Geometry: final body of the model. Coordinates: model frame, mm. A direction names the side the tool comes from. Give positions to 0.01 mm unless a question says otherwise; leave off trailing zeros. Write each loop counter-clockwise with the first axis right and the second up, starting at its lowest first coordinate (ties: lowest second). Pieces come first, ordered by that corner, then holes. Notation, with made-up numbers: M -3.75,6 L 11.25,6 A28 ccw 11.25,28 Z; hole C -9.75,53 d1. An arc over 180 degrees is marked long. Use a Markdown table: item, result. Add a question column.
1) Section B-B on z = -70.5. Return the cut outline in (x, y).
2) Section D-D on y = 26. Return the cut outline in (x, z), then the cut area to 3 significant figures.
3) Pin query (flat end, axial travel): pin 1 (3 mm diameter, centred on x = 128, y = 3.5, fed in from +Z); pin 2 (5 mm diameter, centred on y = 13, z = -29.5, fed in from +X); pin 3 (2 mm diameter, centred on y = 60, z = -17.5, fed in from -X); pin 4 (11 mm diameter, centred on x = 157.5, y = 5, fed in from -Z). Return the tip coordinate at first contact, or that it passes through.
4) Line query: line 1 (X direction, y = 14, z = 0); line 2 (Z direction, x = 198, y = 66.5); line 3 (X direction, y = 4.5, z = 0). Output: solid intervals per line, ascending.
5) Section A-A on x = 0. State how many separate pieces and enclosed holes the cut face has, then the cut area to 3 significant figures.
6) Set-up query: faces 5 (the flat face through (198, 53.3, -11)), 6 (the flat face through (214, 72, 0)), 7 (the flat face through (217.05, 62, 0)), 8 (the cylindrical face through (223.3, 4.93, -3.06)), 9 (the cylindrical face through (-46.245, 14.93, -60.311)). Return all of +Z, -Z, +X, -X, +Y, -Y with unobstructed straight access to the full face (end or side cutting, diameter ignored); none if empty.
7) Draft query along Y for faces 1 (the flat face through (187, 80, 0)), 2 (the flat face through (-57.5, 20, 19)), 3 (the flat face through (190, 63, -15)), 4 (the cylindrical face through (-66.284, 5.07, 2.688)). Return one class per face: +Y half, -Y half, draft (parallel to the pull), parting line (faces both ways), or undercut.
8) Section C-C on x = -70.5. Return the cut outline in (y, z).
```python
from build123d import *

# Parameters (mm, degrees)
CROQUIS1_R                   = 50
CROQUIS1_R_2                 = 23.5
SALIENTE_EXTRUIR1_DEPTH      = 10
REDONDEO1_R                  = 70
CROQUIS2_R                   = 81
CROQUIS2_R_2                 = 76
SALIENTE_EXTRUIR2_DEPTH      = 10
CROQUIS8_W                   = 74
CROQUIS8_H                   = 10
SALIENTE_EXTRUIR4_DEPTH      = 10
CROQUIS9_W                   = 74
CROQUIS9_H                   = 10
SALIENTE_EXTRUIR5_DEPTH      = 80
CROQUIS10_W                  = 74
CROQUIS10_H                  = 10
SALIENTE_EXTRUIR6_DEPTH      = 75
REDONDEO3_R                  = 2
REDONDEO4_R                  = 2
REDONDEO5_R                  = 2
REDONDEO6_R                  = 2
CROQUIS12_R                  = 65
CROQUIS12_R_2                = 60
SALIENTE_EXTRUIR12_DEPTH     = 10
CROQUIS13_R                  = 5
CORTAR_EXTRUIR1_DEPTH        = 10
SALIENTE_EXTRUIR13_OUTLINE_R = 1.25
SALIENTE_EXTRUIR13_DEPTH     = 26.7
REDONDEO7_R                  = 10
CORTAR_EXTRUIR2_START        = -36.7
CROQUIS15_R                  = 1.25
CORTAR_EXTRUIR2_DEPTH        = 36.7
REDONDEO9_R                  = 2.5
CROQUIS17_W                  = 7
CROQUIS17_H                  = 5
CORTAR_EXTRUIR3_DEPTH        = 26.95
CROQUIS18_W                  = 40.143208987
CROQUIS18_H                  = 75
CORTAR_EXTRUIR4_DEPTH        = 5
REDONDEO10_R                 = 1
REDONDEO11_R                 = 1


# Read off the part's stored shape, not the designer's step: Saliente-Extruir13
with BuildPart() as part:
    # Croquis1 → Saliente-Extruir1 (new body)
    with BuildSketch(Plane(origin=(0, 0, 0), x_dir=(1, 0, 0), z_dir=(0, 1, 0))):
        with BuildLine():
            ThreePointArc((-72.570488149, -44.255217205), (4.131356705, -84.899539997), (76.524505879, -37))
            Line((76.524505879, -37), (237, -37))
            Line((237, -37), (237, 0))
            ThreePointArc((237, 0), (226.162950904, 26.162950904), (200, 37))
            Line((200, 37), (76.524505879, 37))
            ThreePointArc((76.524505879, 37), (4.131356705, 84.899539997), (-72.570488149, 44.255217205))
            Line((-72.570488149, 44.255217205), (-135.143208987, 44.255217205))
            Line((-135.143208987, 44.255217205), (-135.143208987, -44.255217205))
            Line((-135.143208987, -44.255217205), (-72.570488149, -44.255217205))
        make_face()
        with Locations(Location((0, 0, 0), (0, 0, 270))):
            Circle(CROQUIS1_R, mode=Mode.SUBTRACT)
        with Locations(Location((200, 0, 0), (0, 0, 270))):
            Circle(CROQUIS1_R_2, mode=Mode.SUBTRACT)
    extrude(amount=SALIENTE_EXTRUIR1_DEPTH)

    # Redondeo1
    redondeo1_edges = [part.edges().sort_by_distance(p)[0] for p in [
        (76.524505879, 5, 37),
        (-72.570488149, 5, 44.255217205),
        (-72.570488149, 5, -44.255217205),
        (76.524505879, 5, -37),
    ]]
    fillet(redondeo1_edges, radius=REDONDEO1_R)

    # Croquis2 → Saliente-Extruir2 (add)
    with BuildSketch(Plane(origin=(0, 10, 0), x_dir=(1, 0, 0), z_dir=(0, 1, 0))):
        with Locations(Location((0, 0, 0), (0, 0, 270))):
            Circle(CROQUIS2_R)
        with Locations(Location((0, 0, 0), (0, 0, 270))):
            Circle(CROQUIS2_R_2, mode=Mode.SUBTRACT)
    extrude(amount=SALIENTE_EXTRUIR2_DEPTH)

    # Croquis8 → Saliente-Extruir4 (add)
    with BuildSketch(Plane.XY.offset(37)):
        with Locations((200, 5)):
            Rectangle(CROQUIS8_W, CROQUIS8_H)
    extrude(amount=SALIENTE_EXTRUIR4_DEPTH)

    # Croquis9 → Saliente-Extruir5 (add)
    with BuildSketch(Plane(origin=(0, 10, 0), x_dir=(1, 0, 0), z_dir=(0, 1, 0))):
        with Locations((200, -42)):
            Rectangle(CROQUIS9_W, CROQUIS9_H)
    extrude(amount=SALIENTE_EXTRUIR5_DEPTH)

    # Croquis10 → Saliente-Extruir6 (add)
    with BuildSketch(Plane(origin=(0, 0, 37), x_dir=(-1, 0, 0), z_dir=(0, 0, -1))):
        with Locations((-200, 85)):
            Rectangle(CROQUIS10_W, CROQUIS10_H)
    extrude(amount=SALIENTE_EXTRUIR6_DEPTH)

    # Redondeo3
    redondeo3_edges = [part.edges().sort_by_distance(p)[0] for p in [
        (200, 10, 37),
    ]]
    fillet(redondeo3_edges, radius=REDONDEO3_R)

    # Redondeo4
    redondeo4_edges = [part.edges().sort_by_distance(p)[0] for p in [
        (200, 80, 37),
    ]]
    fillet(redondeo4_edges, radius=REDONDEO4_R)

    # Redondeo5
    redondeo5_edges = [part.edges().sort_by_distance(p)[0] for p in [
        (200, 90, 47),
    ]]
    fillet(redondeo5_edges, radius=REDONDEO5_R)

    # Redondeo6
    redondeo6_edges = [part.edges().sort_by_distance(p)[0] for p in [
        (200, 90, -38),
    ]]
    fillet(redondeo6_edges, radius=REDONDEO6_R)

    # Croquis12 → Saliente-Extruir12 (add)
    with BuildSketch(Plane(origin=(0, 10, 0), x_dir=(1, 0, 0), z_dir=(0, 1, 0))):
        with Locations(Location((0, 0, 0), (0, 0, 270))):
            Circle(CROQUIS12_R)
        with Locations(Location((0, 0, 0), (0, 0, 270))):
            Circle(CROQUIS12_R_2, mode=Mode.SUBTRACT)
    extrude(amount=SALIENTE_EXTRUIR12_DEPTH)

    # Croquis13 → Cortar-Extruir1 (cut)
    with BuildSketch(Plane(origin=(0, 10, 0), x_dir=(1, 0, 0), z_dir=(0, 1, 0))):
        with Locations(Location((-70.5, 0, 0), (0, 0, 270))):
            Circle(CROQUIS13_R)
        with Locations(Location((0, 70.5, 0), (0, 0, 270))):
            Circle(CROQUIS13_R)
        with Locations(Location((70.5, 0, 0), (0, 0, 270))):
            Circle(CROQUIS13_R)
        with Locations(Location((0, -70.5, 0), (0, 0, 270))):
            Circle(CROQUIS13_R)
    extrude(amount=-CORTAR_EXTRUIR1_DEPTH, mode=Mode.SUBTRACT)

    # Saliente-Extruir13 outline → Saliente-Extruir13 (add)
    with BuildSketch(Plane.XZ.offset(-80)):
        Polygon((163, -10), (163, -15), (217.05, -15), (217.05, 15), (163, 15), (163, 10), (210.05, 10), (210.05, -10), align=None)
        with Locations((214.55, -4.95)):
            Circle(SALIENTE_EXTRUIR13_OUTLINE_R, mode=Mode.SUBTRACT)
        with Locations((214.55, 4.95)):
            Circle(SALIENTE_EXTRUIR13_OUTLINE_R, mode=Mode.SUBTRACT)
    extrude(amount=SALIENTE_EXTRUIR13_DEPTH)

    # Redondeo7
    redondeo7_edges = [part.edges().sort_by_distance(p)[0] for p in [
        (190.025, 80, -15),
        (190.025, 80, 15),
        (217.05, 80, 0),
    ]]
    fillet(redondeo7_edges, radius=REDONDEO7_R)

    # Croquis15 → Cortar-Extruir2 (cut)
    with BuildSketch(Plane.XZ.offset(-53.3).offset(CORTAR_EXTRUIR2_START)):
        with Locations(Location((214.55, 4.95, 0), (0, 0, 270))):
            Circle(CROQUIS15_R)
        with Locations(Location((214.55, -4.95, 0), (0, 0, 270))):
            Circle(CROQUIS15_R)
    extrude(amount=CORTAR_EXTRUIR2_DEPTH, mode=Mode.SUBTRACT)

    # Redondeo9
    redondeo9_edges = [part.edges().sort_by_distance(p)[0] for p in [
        (190.025, 53.3, 15),
        (190.025, 53.3, -15),
    ]]
    fillet(redondeo9_edges, radius=REDONDEO9_R)

    # Croquis17 → Cortar-Extruir3 (cut)
    with BuildSketch(Plane(origin=(237, 0, 0), x_dir=(0, 0, -1), z_dir=(1, 0, 0))):
        with Locations((0, 74.5)):
            Rectangle(CROQUIS17_W, CROQUIS17_H)
    extrude(amount=-CORTAR_EXTRUIR3_DEPTH, mode=Mode.SUBTRACT)

    # Croquis18 → Cortar-Extruir4 (cut)
    with BuildSketch(Plane(origin=(0, 10, 0), x_dir=(1, 0, 0), z_dir=(0, 1, 0))):
        with Locations((-111.071604494, 0.005217205)):
            Rectangle(CROQUIS18_W, CROQUIS18_H)
    extrude(amount=-CORTAR_EXTRUIR4_DEPTH, mode=Mode.SUBTRACT)

    # Redondeo10
    redondeo10_edges = [part.edges().sort_by_distance(p)[0] for p in [
        (-91, 7.5, -37.505217205),
        (-111.071604493, 5, 37.494782795),
        (-91, 7.5, 37.494782795),
        (-131.143208987, 5, -0.005217205),
        (-131.143208987, 7.5, 37.494782795),
        (-131.143208987, 7.5, -37.505217205),
        (-91, 5, -0.005217205),
        (-111.071604493, 5, -37.505217205),
    ]]
    fillet(redondeo10_edges, radius=REDONDEO10_R)

    # Redondeo11
    redondeo11_edges = [part.edges().sort_by_distance(p)[0] for p in [
        (-135.143208987, 5, -44.255217205),
        (-135.143208987, 5, 44.255217205),
    ]]
    fillet(redondeo11_edges, radius=REDONDEO11_R)


solid = part.part
```
Found:
| question | item | result |
|---|---|---|
| 1 | outline | M -47.48,0 L -5,0 L -5,10 L -28.39,10 L -28.39,20 L -39.88,20 L -39.88,10 L -47.48,10 Z; M 5,0 L 47.48,0 L 47.48,10 L 39.88,10 L 39.88,20 L 28.39,20 L 28.39,10 L 5,10 Z |
| 2 | outline | M 163,37 L 237,37 L 237,47 L 163,47 Z |
| 2 | area | 740 mm² |
| 3 | pin 1 | z = 37 |
| 3 | pin 2 | x = 76.37 |
| 3 | pin 3 | through |
| 3 | pin 4 | z = -37 |
| 4 | line 1 | -81 to -76, -65 to -60, 60 to 65, 76 to 81 |
| 4 | line 2 | -15 to -10, 10 to 15, 37 to 47 |
| 4 | line 3 | -135.14 to -75.5, -65.5 to -50, 50 to 65.5, 75.5 to 176.5, 223.5 to 237 |
| 5 | separate pieces | 4 |
| 5 | enclosed holes | 0 |
| 5 | area | 700 mm² |
| 6 | face 5 | -Z, +X, -X |
| 6 | face 6 | +X, -X |
| 6 | face 7 | -Z, +X, -Y |
| 6 | face 8 | -Y |
| 6 | face 9 | +Y |
| 7 | face 1 | undercut |
| 7 | face 2 | +Y half |
| 7 | face 3 | undercut |
| 7 | face 4 | draft |
| 8 | outline | M 0,-53.2 L 10,-53.2 L 10,-39.88 L 20,-39.88 L 20,-28.39 L 10,-28.39 L 10,-5 L 0,-5 Z; M 0,5 L 10,5 L 10,28.39 L 20,28.39 L 20,39.88 L 10,39.88 L 10,53.2 L 0,53.2 Z |
